```python
from build123d import *

# Parameters (mm, degrees)
PAD_DEPTH       = 10
SKETCH001_R     = 1.6
POCKET_DEPTH    = 17.001
POCKET001_DEPTH = 2.5
FILLET_R        = 1.5
FILLET001_R     = 1
CHAMFER_SIZE    = 1


with BuildPart() as part:
    # Sketch → Pad (new body)
    with BuildSketch(Plane.XY):
        Polygon((-12.5, -8.5), (-12.5, 3.5), (12.5, 3.5), (12.5, -8.5), (22.5, -8.5), (22.5, 8.5), (-22.5, 8.5), (-22.5, -8.5), align=None)
    extrude(amount=PAD_DEPTH)

    # Sketch001 (on Face4 of Pad) → Pocket (cut, through all)
    with BuildSketch(Plane.XZ.offset(8.5)):
        with Locations((-17.5, 5)):
            Circle(SKETCH001_R)
        with Locations((17.5, 5)):
            Circle(SKETCH001_R)
    extrude(amount=-POCKET_DEPTH, mode=Mode.SUBTRACT)

    # Sketch002 (on Face11 of Pocket) → Pocket001 (cut)
    with BuildSketch(Plane(origin=(0, 8.5, 0), x_dir=(-1, 0, 0), z_dir=(0, 1, 0))):
        Polygon((-17.5, 8.233162), (-20.3, 6.616581), (-20.3, 3.383419), (-17.5, 1.766838), (-14.7, 3.383419), (-14.7, 6.616581), align=None)
        Polygon((17.5, 8.233162), (14.7, 6.616581), (14.7, 3.383419), (17.5, 1.766838), (20.3, 3.383419), (20.3, 6.616581), align=None)
    extrude(amount=-POCKET001_DEPTH, mode=Mode.SUBTRACT)

    # Fillet
    fillet_edges = [part.edges().sort_by_distance(p)[0] for p in [
        (0, 8.5, 0),
        (0, 8.5, 10),
        (-22.5, 8.5, 5),
        (22.5, 8.5, 5),
    ]]
    fillet(fillet_edges, radius=FILLET_R)

    # Fillet001
    fillet001_edges = [part.edges().sort_by_distance(p)[0] for p in [
        (-12.5, -2.5, 0),
        (-12.5, -2.5, 10),
        (-22.5, -0.75, 0),
        (-22.5, -0.75, 10),
        (12.5, -2.5, 10),
        (12.5, -2.5, 0),
        (22.5, -0.75, 0),
        (22.5, -0.75, 10),
    ]]
    fillet(fillet001_edges, radius=FILLET001_R)

    # Chamfer
    chamfer_edges = [part.edges().sort_by_distance(p)[0] for p in [
        (0, 3.5, 0),
        (0, 3.5, 10),
    ]]
    chamfer(chamfer_edges, length=CHAMFER_SIZE)


solid = part.part
```
Geometry check sheet. Reference: the model listing, model coordinates, mm. A direction names the side the tool comes from. Give positions to 0.01 mm unless a question says otherwise; leave off trailing zeros. Order: outer loops, then holes, each group sorted by start corner. A loop starts at its lowest first (then second) coordinate and runs counter-clockwise, first axis right, second up. Notation, with made-up numbers: (-17, -3.5) - (36, -3.5) arc R16 cw to (36, 21.5) - close; hole circle Ø9 at (65, -4.75). An arc over 180 degrees is marked (long way). Answer in a Markdown table with one row per item. Add a question column.
Q1. Material ranges on probe 1 along X at (y, z) = (6.75, 4.5); probe 2 along X at (y, z) = (-7, 5.75); probe 3 along Z at (x, y) = (17.5, -3), recorded low to high. Write a range as from..to.
Q2. Tool access check on faces 5 (the flat face through (19, 6, 4)), 6 (the flat face through (-12.5, -3, 5)), 7 (the cylindrical face through (12.785, -2.091, 9.699)), 8 (the cylindrical face through (12.801, -2.091, 0.285)). Record the directions out of +Z, -Z, +X, -X, +Y, -Y that give a thin tool (end or side, any length) a straight path to the whole face; none if there is none.
Q3. Cross-section at A-A, the plane y = -3. Enter the section's corners in (x, z).
Q4. Cross-section at B-B, the plane z = 5. Enter the section's corners in (x, y).
Q5. Cross-section at C-C, the plane x = 7. Enter the section's corners in (y, z), then the cut area to 3 significant figures.
Q6. Gauge pin test, flat ends, axial feed: pin 1 (6 mm diameter, centred on x = -17, z = 6.5, fed in from +Y); pin 2 (3.5 mm diameter, centred on x = 17.5, z = 5, fed in from +Y). Record the tip position at first contact, or that the pin passes through.
Q7. Mould release check, pull along Z, two halves, no side actions. Record for faces 1 (the cylindrical face through (-22.215, -0.859, 9.699)), 2 (the flat face through (-16.08, 7.268, 2.586)), 3 (the flat face through (18.88, 7.268, 7.436)), 4 (the flat face through (-22.5, -1, 5)): pulls with the +Z half, pulls with the -Z half, needs draft (parallel to the pull), parting line crosses it, or undercut.
Q8. Cross-section at D-D, the plane x = -18.5. Enter the section's corners in (y, z), then the cut area to 3 significant figures.
Check values:
| question | item | result |
|---|---|---|
| 1 | probe 1 | x = -22.5..-20.3, -14.7..14.7, 20.3..22.5 |
| 1 | probe 2 | x = -22.5..-18.91, -16.09..-12.5, 12.5..16.09, 18.91..22.5 |
| 1 | probe 3 | z = 0..3.4, 6.6..10 |
| 2 | face 5 | +Y |
| 2 | face 6 | +Z, -Z, -Y |
| 2 | face 7 | +Z, -Y |
| 2 | face 8 | -Z, -Y |
| 3 | outline | (-22.5, 1) arc R1 ccw to (-21.5, 0) - (-13.5, 0) arc R1 ccw to (-12.5, 1) - (-12.5, 9) arc R1 ccw to (-13.5, 10) - (-21.5, 10) arc R1 ccw to (-22.5, 9) - close; (12.5, 1) arc R1 ccw to (13.5, 0) - (21.5, 0) arc R1 ccw to (22.5, 1) - (22.5, 9) arc R1 ccw to (21.5, 10) - (13.5, 10) arc R1 ccw to (12.5, 9) - close; hole circle Ø3.2 at (-17.5, 5); hole circle Ø3.2 at (17.5, 5) |
| 4 | outline | (-22.5, -8.5) - (-19.1, -8.5) - (-19.1, 6) - (-20.3, 6) - (-20.3, 8.5) - (-21, 8.5) arc R1.5 ccw to (-22.5, 7) - close; (-15.9, -8.5) - (-12.5, -8.5) - (-12.5, 3.5) - (12.5, 3.5) - (12.5, -8.5) - (15.9, -8.5) - (15.9, 6) - (14.7, 6) - (14.7, 8.5) - (-14.7, 8.5) - (-14.7, 6) - (-15.9, 6) - close; (19.1, -8.5) - (22.5, -8.5) - (22.5, 7) arc R1.5 ccw to (21, 8.5) - (20.3, 8.5) - (20.3, 6) - (19.1, 6) - close |
| 5 | outline | (3.5, 1) - (4.5, 0) - (7, 0) arc R1.5 ccw to (8.5, 1.5) - (8.5, 8.5) arc R1.5 ccw to (7, 10) - (4.5, 10) - (3.5, 9) - close |
| 5 | area | 48.0 mm^2 |
| 6 | pin 1 | stops at y = 8.5 |
| 6 | pin 2 | stops at y = 6 |
| 7 | face 1 | pulls with the +Z half |
| 7 | face 2 | undercut |
| 7 | face 3 | undercut |
| 7 | face 4 | needs draft |
| 8 | outline | (-8.5, 0) - (7, 0) arc R1.5 ccw to (8.5, 1.5) - (8.5, 2.34) - (6, 2.34) - (6, 3.75) - (-8.5, 3.75) - close; (-8.5, 6.25) - (6, 6.25) - (6, 7.66) - (8.5, 7.66) - (8.5, 8.5) arc R1.5 ccw to (7, 10) - (-8.5, 10) - close |
| 8 | area | 120 mm^2 |
